Can you work these out from the model? Positions are in its coordinate system, mm. Face numbers are marked on the shaded views. Give positions to 0.01 mm unless a question says otherwise; leave off trailing zeros. Order: outer loops, then holes, each group sorted by start corner. A loop starts at its lowest first (then second) coordinate and runs counter-clockwise, first axis right, second up. Notation, with made-up numbers: M 89,36 L 141,36 A17 ccw 141,41 Z; hole C 25.25,-24 d8. An arc over 180 degrees is marked long. Use a Markdown table: item, result. Add a question column.
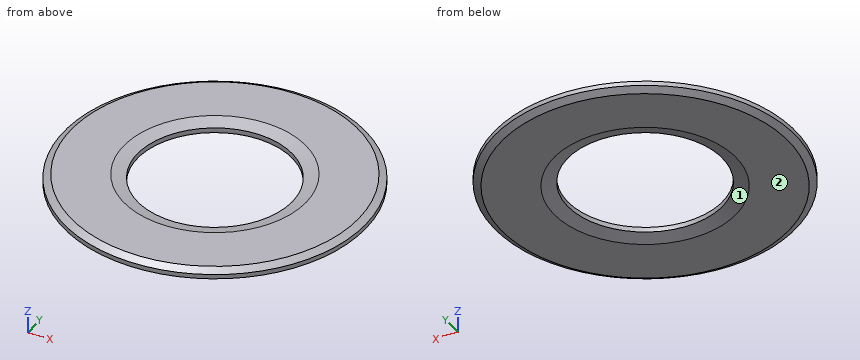
from build123d import *
from OCP.BRepFilletAPI import BRepFilletAPI_MakeChamfer

# Parameters (mm, degrees)
BOSS_EXTRUDE1_DEPTH      = 0.39624
BOSS_EXTRUDE1_DEPTH_BACK = 0.39624
SKETCH3_R                = 9.525
SKETCH3_R_2              = 4.8895
CHAMFER1_SIZE            = 0.254
CHAMFER1_SIZE2           = 0.439940905
CHAMFER2_SIZE            = 0.828943919


with BuildPart() as part:
    # Sketch3 → Boss-Extrude1 (new, two sides: drawn at the far end of the back side and taken through both)
    with BuildSketch(Plane.XY.offset(-BOSS_EXTRUDE1_DEPTH_BACK)):
        Circle(SKETCH3_R)
        Circle(SKETCH3_R_2, mode=Mode.SUBTRACT)
    extrude(amount=BOSS_EXTRUDE1_DEPTH + BOSS_EXTRUDE1_DEPTH_BACK)

    # Chamfer1: one chamfer whose edges measure the first distance from different faces: ONE call of the kernel's chamfer builder (chamfer() names one face for all edges)
    chamfer1_edges_1 = [part.edges().sort_by_distance(p)[0] for p in [
        (-9.525, 0, 0.39624),
    ]]
    chamfer1_side_1 = [part.faces().sort_by_distance(p)[0] for p in [
        (-9.525, 0, 0.19812),
    ]]
    chamfer1_edges_2 = [part.edges().sort_by_distance(p)[0] for p in [
        (-9.525, 0, -0.39624),
    ]]
    chamfer1_side_2 = [part.faces().sort_by_distance(p)[0] for p in [
        (-9.525, 0, -0.19812),
    ]]
    chamfer1 = BRepFilletAPI_MakeChamfer(part.part.solid().wrapped)
    for e in chamfer1_edges_1:
        chamfer1.Add(CHAMFER1_SIZE, CHAMFER1_SIZE2, e.wrapped, chamfer1_side_1[0].wrapped)  # the first distance lies on this face
    for e in chamfer1_edges_2:
        chamfer1.Add(CHAMFER1_SIZE, CHAMFER1_SIZE2, e.wrapped, chamfer1_side_2[0].wrapped)  # the first distance lies on this face
    add(Compound.cast(chamfer1.Shape()), mode=Mode.REPLACE)

    # Sketch4 → Cut-Revolve1 (revolve, cut)
    with BuildSketch(Plane(origin=(0, 0, 0), x_dir=(0, 0, -1), z_dir=(1, 0, 0)), mode=Mode.PRIVATE) as cut_revolve1_sk:
        with BuildLine():
            Line((-0.39624, 4.8387), (-0.39624, 4.9403))
            ThreePointArc((-0.39624, 4.9403), (0, 4.8895), (0.39624, 4.9403))
            Line((0.39624, 4.9403), (0.39624, 4.8387))
            Line((0.39624, 4.8387), (-0.39624, 4.8387))
        make_face()
    revolve(cut_revolve1_sk.sketch.rotate(Axis((0, 0, 0.39624), (0, 0, -1)), 90), axis=Axis((0, 0, 0.39624), (0, 0, -1)), mode=Mode.SUBTRACT)

    # Chamfer2
    # the kernel refuses this chamfer: 0.828943919, 0.254 mm, written as the material it takes off along each edge
    with BuildSketch(Plane(origin=(0, 0, -0.39624), x_dir=(1, 0, 0), z_dir=(0, 1, 0))) as chamfer2_piece_1:
        with BuildLine():
            Line((4.9403 + CHAMFER2_SIZE, 0), (4.897291135, -0.239987219))
            ThreePointArc((4.897291135, -0.239987219), (4.91289484, -0.126153132), (4.9403, 0))
            Line((4.9403, 0), (4.9403 + CHAMFER2_SIZE, 0))
        make_face()
    revolve(axis=Axis((0, 0, -0.39624), (0, 0, -1)), mode=Mode.SUBTRACT)
    with BuildSketch(Plane(origin=(0, 0, 0.39624), x_dir=(1, 0, 0), z_dir=(0, 1, 0))) as chamfer2_piece_2:
        with BuildLine():
            Line((4.9403 + CHAMFER2_SIZE, 0), (4.897291135, 0.239987219))
            ThreePointArc((4.897291135, 0.239987219), (4.91289484, 0.126153132), (4.9403, 0))
            Line((4.9403, 0), (4.9403 + CHAMFER2_SIZE, 0))
        make_face()
    revolve(axis=Axis((0, 0, 0.39624), (0, 0, -1)), mode=Mode.SUBTRACT)


solid = part.part
1. If we section it at A-A, the plane y = 0: List the corners of the cut face in (x, z) for me (3 decimals), then the cut area to 3 significant figures.
2. Will these pins go through, and if not, where does the flat tip stop? pin 1 (6 mm diameter, centred on x = -0.5, y = -2.5, fed in from +Z); pin 2 (10 mm diameter, centred on x = 6, y = 7, fed in from -Z).
3. We'd pull the mould along Y, two halves only. Please class the marked faces 1 and 2: +Y half, -Y half, draft (parallel to the pull), parting line (faces both ways), or undercut.
4. I need wall thicknesses on L1, parallel to X at y = -4.5, z = 0.1; L2, parallel to Y at x = 3.5, z = 0; L3, parallel to X at y = 8.75, z = 0.1. Which ranges of each line are inside material? Lowest first, please. Write a range as [from, to].
Geometry results:
| question | item | result |
|---|---|---|
| 1 | outline | M -9.525,-0.142 L -9.085,-0.396 L -5.769,-0.396 L -4.897,-0.156 A1.571 ccw -4.897,0.156 L -5.769,0.396 L -9.085,0.396 L -9.525,0.142 Z; M 4.897,-0.156 L 5.769,-0.396 L 9.085,-0.396 L 9.525,-0.142 L 9.525,0.142 L 9.085,0.396 L 5.769,0.396 L 4.897,0.156 A1.571 ccw Z |
| 1 | area | 6.70 mm^2 |
| 2 | pin 1 | stops at z = 0.34 |
| 2 | pin 2 | stops at z = -0.4 |
| 3 | face 1 | undercut |
| 3 | face 2 | draft |
| 4 | L1 | x = [-8.39, -1.92], [1.92, 8.39] |
| 4 | L2 | y = [-8.86, -3.41], [3.41, 8.86] |
| 4 | L3 | x = [-3.76, 3.76] |
